Build history of the part. All positions in model axes, mm. Give positions to 0.01 mm unless a question says otherwise; leave off trailing zeros. Order: outer loops, then holes, each group sorted by start corner. A loop starts at its lowest first (then second) coordinate and runs counter-clockwise, first axis right, second up. Notation, with made-up numbers: (75.5, 82) -> (79.5, 82) arc R15 ccw to (79.5, 92) -> close; hole circle Ø10 at (54, 58.5). An arc over 180 degrees is marked (long way). One line per item, written item: value. Start each with the question number.
(1) Probe line 1 (X direction, y = 12, z = -17.9); line 2 (X direction, y = 120, z = 0); line 3 (Z direction, x = 0.25, y = 102.5). List the from-to ranges inside material, lowest first.
(2) Saw through at B-B on y = 144.5. Give the cut face in (x, z).
(3) Saw through at A-A on z = 14. Give the cut face in (x, y).
(4) Pin check, flat tips, straight feed: pin 1 (2 mm diameter, centred on x = 0, z = -8.5, fed in from +Y); pin 2 (5 mm diameter, centred on x = 3.5, y = 244.5, fed in from -Z); pin 3 (0.6 mm diameter, centred on x = -4, y = 241.5, fed in from +Z); pin 4 (4.5 mm diameter, centred on x = 3, z = 0, fed in from -Y). Stop position of each tip, or through.
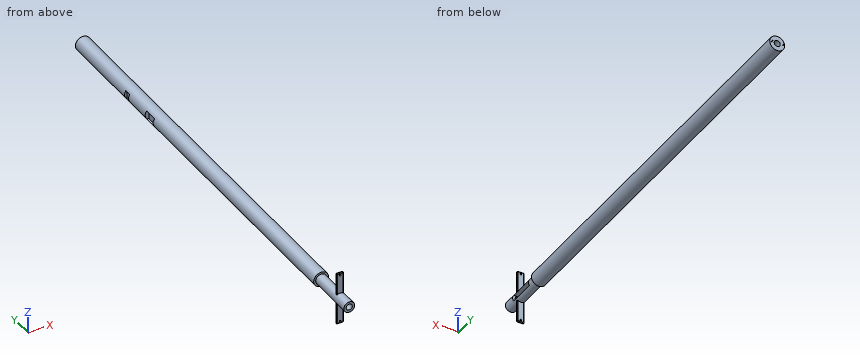
```python
from build123d import *

# Parameters (mm, degrees)
SWEEP3_PROFILE_R         = 4
SWEEP4_PROFILE_R         = 5.5
SKETCH45_R               = 2.25
CUT_EXTRUDE2_DEPTH       = 337.377466094
SWEEP5_PROFILE_R         = 0.25
SWEEP6_PROFILE_R         = 0.25
SKETCH72_W               = 4.5
SKETCH72_H               = 20
CUT_EXTRUDE6_DEPTH       = 20
BOSS_EXTRUDE1_DEPTH      = 2.5
BOSS_EXTRUDE1_DEPTH_BACK = 2.5
BOSS_EXTRUDE3_DEPTH      = 2.5
BOSS_EXTRUDE3_DEPTH_BACK = 2.5
SKETCH76_4_W             = 16.5
SKETCH76_4_H             = 1.4
SKETCH77_R               = 0.612238256
CUT_EXTRUDE7_DEPTH       = 20
FILLET1_R                = 0.5
CUT_EXTRUDE9_DEPTH       = 3
CUT_EXTRUDE9_DEPTH_BACK  = 3


with BuildPart() as part:
    # Sweep3: sweep along a path in Sketch31
    with BuildLine(Plane.XY) as sweep3_path:
        Line((0, 0), (0, 35.470165431))
    # Sweep3 profile (on start of the path) → Sweep3 (sweep)
    with BuildSketch(Plane.ZX):
        Circle(SWEEP3_PROFILE_R)
    sweep(path=sweep3_path.line)

    # Sweep4: sweep along a path in Sketch38
    with BuildLine(Plane.XY) as sweep4_path:
        Line((0, 35.470165431), (0, 336.287525335))
    # Sweep4 profile (on start of the path) → Sweep4 (sweep)
    with BuildSketch(Plane.ZX.offset(35.470165431)):
        Circle(SWEEP4_PROFILE_R)
    sweep(path=sweep4_path.line)

    # Sketch45 → Cut-Extrude2 (cut, through all)
    with BuildSketch(Plane(origin=(0, 0, 0), x_dir=(1, 0, 0), z_dir=(0, 1, 0))):
        with Locations(Location((0, 0, 0), (0, 0, 270))):
            Circle(SKETCH45_R)
    extrude(amount=CUT_EXTRUDE2_DEPTH, mode=Mode.SUBTRACT)

    # Sweep5: sweep along a curve in space
    with BuildLine() as sweep5_path:
        Line((4.125, 336.287525335, 5.531e-06), (4.125, 337.787525335, 5.531e-06))
    # Sweep5 profile (on start of the path) → Sweep5 (sweep)
    with BuildSketch(Plane(origin=(4.125, 336.287525335, 5.531e-06), x_dir=(0, 0, 1), z_dir=(0, 1, 0))):
        Circle(SWEEP5_PROFILE_R)
    sweep(path=sweep5_path.line)

    # Sweep6: sweep along a curve in space
    with BuildLine() as sweep6_path:
        Line((-4.125, 336.287525335, 9.31e-07), (-4.125, 337.787525335, 9.31e-07))
    # Sweep6 profile (on start of the path) → Sweep6 (sweep)
    with BuildSketch(Plane(origin=(-4.125, 336.287525335, 9.31e-07), x_dir=(0, 0, 1), z_dir=(0, 1, 0))):
        Circle(SWEEP6_PROFILE_R)
    sweep(path=sweep6_path.line)

    # Sketch72 → Cut-Extrude6 (cut)
    with BuildSketch(Plane(origin=(0, 0, 0), x_dir=(0, 0, -1), z_dir=(1, 0, 0))):
        with Locations((-0.068000409, 19.236124066)):
            Rectangle(SKETCH72_W, SKETCH72_H)
    extrude(amount=CUT_EXTRUDE6_DEPTH, mode=Mode.SUBTRACT)

    # Sketch76 → Boss-Extrude1 (add, two sides: drawn at the far end of the back side and taken through both)
    with BuildSketch(Plane(origin=(0, 0, 0), x_dir=(0, 0, -1), z_dir=(1, 0, 0)).offset(-BOSS_EXTRUDE1_DEPTH_BACK)):
        Polygon((-3, 12.070165431), (-3, 12.770165431), (-19.5, 12.770165431), (-19.5, 12.370165431), (-19.5, 11.370165431), (-3, 11.370165431), align=None)
    extrude(amount=BOSS_EXTRUDE1_DEPTH + BOSS_EXTRUDE1_DEPTH_BACK)

    # Sketch76_4 → Boss-Extrude3 (add, two sides: drawn at the far end of the back side and taken through both)
    with BuildSketch(Plane(origin=(0, 0, 0), x_dir=(0, 0, -1), z_dir=(1, 0, 0)).offset(-BOSS_EXTRUDE3_DEPTH_BACK)):
        with Locations((11.25, 12.070165431)):
            Rectangle(SKETCH76_4_W, SKETCH76_4_H)
    extrude(amount=BOSS_EXTRUDE3_DEPTH + BOSS_EXTRUDE3_DEPTH_BACK)

    # Sketch77 → Cut-Extrude7 (cut)
    with BuildSketch(Plane(origin=(0, 0, 0), x_dir=(1, 0, 0), z_dir=(0, 1, 0))):
        with Locations(Location((0, 17.9, 0), (0, 0, 90))):
            Circle(SKETCH77_R)
        with Locations(Location((0, -17.9, 0), (0, 0, 90))):
            Circle(SKETCH77_R)
    extrude(amount=CUT_EXTRUDE7_DEPTH, mode=Mode.SUBTRACT)

    # Fillet1
    fillet1_edges = [part.edges().sort_by_distance(p)[0] for p in [
        (0, 12.770165431, 19.5),
        (2.5, 12.770165431, 11.3112495),
        (-2.5, 11.370165431, 11.3112495),
        (0, 11.370165431, 19.5),
        (2.5, 12.070165431, 19.5),
        (-2.5, 12.770165431, 11.3112495),
        (2.5, 11.370165431, 11.3112495),
        (0, 11.370165431, -19.5),
        (2.5, 11.370165431, -11.3112495),
        (2.5, 12.770165431, -11.3112495),
        (0, 12.770165431, -19.5),
        (-2.5, 12.770165431, -11.3112495),
        (-2.5, 11.370165431, -11.3112495),
        (2.5, 12.070165431, -19.5),
    ]]
    fillet(fillet1_edges, radius=FILLET1_R)

    # Sketch81 → Cut-Extrude9 (cut, two sides: drawn at the far end of the back side and taken through both)
    with BuildSketch(Plane.XY.offset(-CUT_EXTRUDE9_DEPTH_BACK)):
        Polygon((-3.370825875, 247.178368204), (-51.601612029, 269.074039778), (-3.592025731, 269.074039778), (-3.592025731, 274.074039778), (-49.327088533, 274.074039778), (-55.247485048, 261.387475818), (-3.370825875, 237.178368204), align=None)
    extrude(amount=CUT_EXTRUDE9_DEPTH + CUT_EXTRUDE9_DEPTH_BACK, mode=Mode.SUBTRACT)


solid = part.part
```
Results below:
1. line 1: x = -2.5 to -0.61, 0.61 to 2.5
1. line 2: x = -5.5 to -2.25, 2.25 to 5.5
1. line 3: z = -5.49 to -2.24, 2.24 to 5.49
2. outline: circle Ø11 at (0, 0); hole circle Ø4.5 at (0, 0)
3. outline: (-2.5, 11.87) arc R0.5 ccw to (-2, 11.37) -> (2, 11.37) arc R0.5 ccw to (2.5, 11.87) -> (2.5, 12.27) arc R0.5 ccw to (2, 12.77) -> (-2, 12.77) arc R0.5 ccw to (-2.5, 12.27) -> close
4. pin 1: stops at y = 12.77
4. pin 2: stops at z = -5.41
4. pin 3: stops at z = 4.07
4. pin 4: stops at y = 0
